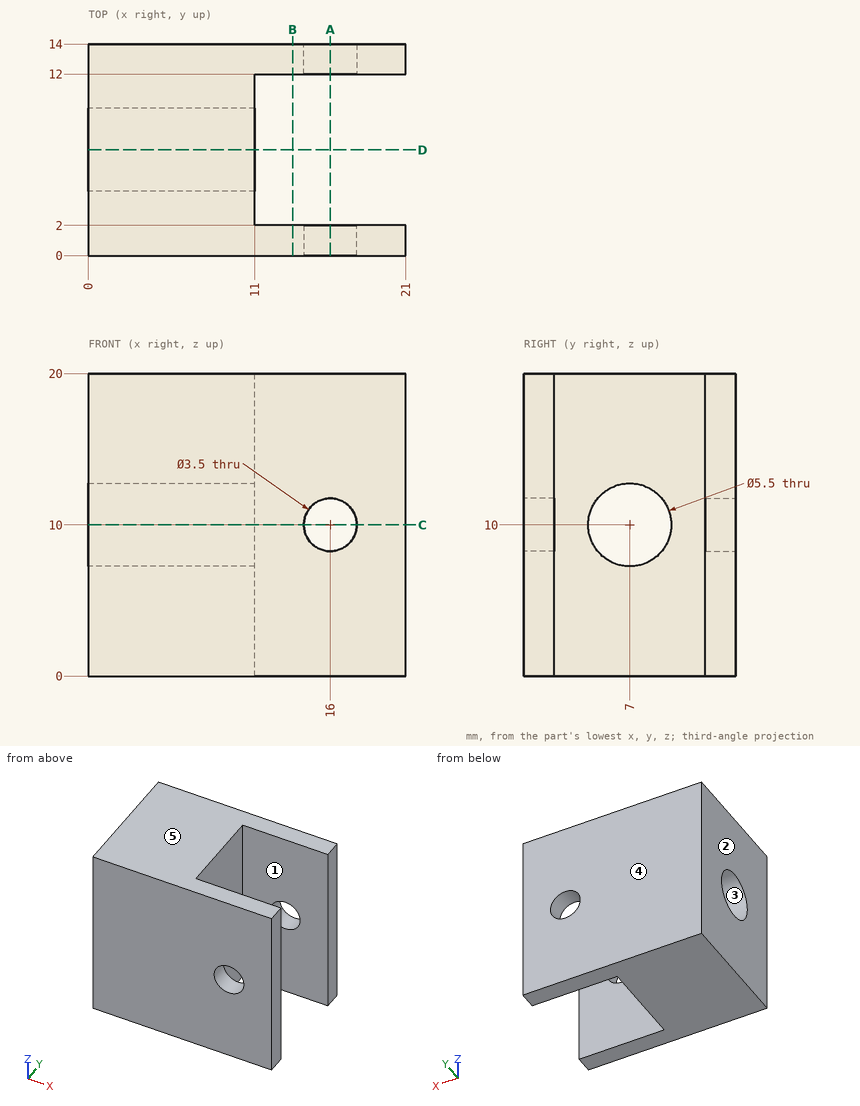
Design review of the part shown in the three views and the two pictorial views. Dimensions are in mm from the part's minimum x, y and z. A direction names the side the tool comes from. Round coordinates to 2 decimals unless told otherwise and drop trailing zeros. Write each loop counter-clockwise with the first axis right and the second up, starting at its lowest first coordinate (ties: lowest second). Pieces come first, ordered by that corner, then holes.
Item 1: Consider section B-B on x = 13.5. Give the boundary of the cut face in (y, z).
Item 2: Draft analysis for pull direction Z (two halves, no side actions). For the marked faces 3, 4 and 5, state which applies: released by +Z, released by -Z, zero draft, split by the parting line, or undercut.
Item 3: For the marked faces 1 and 2, list the 3-axis set-ups (+Z, -Z, +X, -X, +Y, -Y) from which the entire face can be reached by the end or side of a thin tool; tool diameter is ignored.
Item 4: Consider section D-D on y = 7. Give the boundary of the cut face in (x, z), and give its area (4 significant figures).
Item 5: Consider section A-A on x = 16. Give the boundary of the cut face in (y, z).
Item 6: Consider section C-C on z = 10. Give the boundary of the cut face in (x, y).
Item 7: Wall thickness on L1, parallel to Y at x = 11.5, z = 17.25; L2, parallel to Y at x = 6.75, z = 10; L3, parallel to Z at x = 16, y = 0.8: over which ranges is each line inside the solid? List them lowest first.
Item 8: For pin 1 Ø3 at (x, z) = (15, 13) entering from -Y; pin 2 Ø3 at (x, z) = (16, 10) entering from +Y; pin 3 Ø6 at (y, z) = (7.5, 11) entering from +X, all flat-tipped, find the tip position at first contact; note any pin that passes through.
Check values:
1. outline: (0, 0) - (2, 0) - (2, 20) - (0, 20) - close; (12, 0) - (14, 0) - (14, 20) - (12, 20) - close
2. face 3: undercut
2. face 4: zero draft
2. face 5: released by +Z
3. face 1: +Z, -Z, +X
3. face 2: +Z, -Z, -X, +Y, -Y
4. outline: (0, 0) - (11, 0) - (11, 7.25) - (0, 7.25) - close; (0, 12.75) - (11, 12.75) - (11, 20) - (0, 20) - close
4. area: 159.5 mm2
5. outline: (0, 0) - (2, 0) - (2, 8.25) - (0, 8.25) - close; (0, 11.75) - (2, 11.75) - (2, 20) - (0, 20) - close; (12, 0) - (14, 0) - (14, 8.25) - (12, 8.25) - close; (12, 11.75) - (14, 11.75) - (14, 20) - (12, 20) - close
6. outline: (0, 0) - (14.25, 0) - (14.25, 2) - (11, 2) - (11, 4.25) - (0, 4.25) - close; (0, 9.75) - (11, 9.75) - (11, 12) - (14.25, 12) - (14.25, 14) - (0, 14) - close; (17.75, 0) - (21, 0) - (21, 2) - (17.75, 2) - close; (17.75, 12) - (21, 12) - (21, 14) - (17.75, 14) - close
7. L1: y = 0 to 2, 12 to 14
7. L2: y = 0 to 4.25, 9.75 to 14
7. L3: z = 0 to 8.25, 11.75 to 20
8. pin 1: stops at y = 0
8. pin 2: passes through
8. pin 3: stops at x = 11
